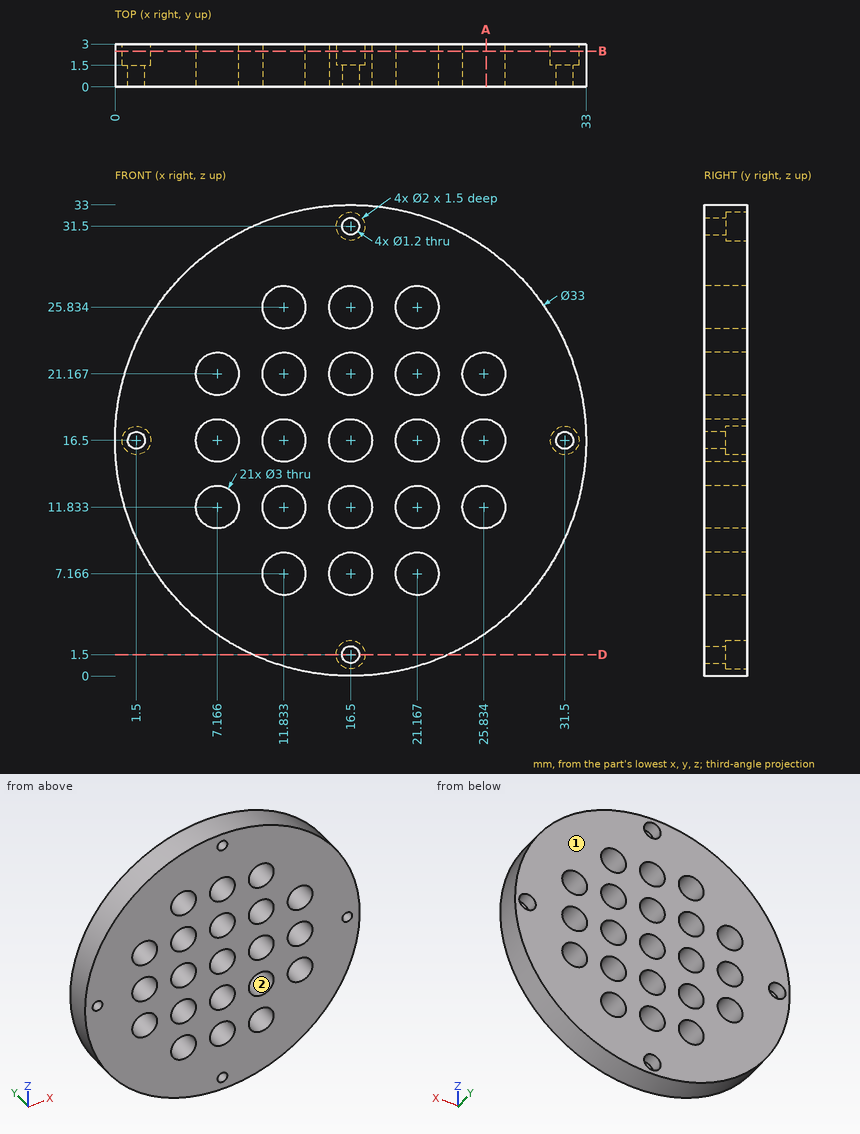
Here's the drawing with two shaded views (mm, measured from the low corner). I have some questions. Round coordinates to 2 decimals unless told otherwise and drop trailing zeros. Loops run counter-clockwise (first coordinate to the right, second up) from the corner with the lowest first, then second, coordinate; pieces in that order, holes last. Notation, with made-up numbers: M 88,-23.75 L 95,-23.75 A16 ccw 95,-0.75 Z; hole C 81,-3 d11. An arc over 180 degrees is marked long. Put each result on its own line as item: value.
Q1. Imagine slicing it at D-D (z = 1.5). Write out the boundary of the cut face in (x, y).
Check result:
outline: M 9.63,0 L 15.9,0 L 15.9,1.5 L 15.5,1.5 L 15.5,3 L 9.63,3 Z; M 17.1,0 L 23.37,0 L 23.37,3 L 17.5,3 L 17.5,1.5 L 17.1,1.5 Z
Q2. Imagine slicing it at B-B (y = 2.5). State how many separate pieces and enclosed holes the cut face has, then the cut area to 3 significant figures.
Check result:
separate pieces: 1
enclosed holes: 25
area: 694 mm2
Q3. Imagine slicing it at A-A (x = 26). Write out the boundary of the cut face in (y, z), then the cut area to 3 significant figures.
Check result:
outline: M 0,3.01 L 3,3.01 L 3,10.34 L 0,10.34 Z; M 0,13.32 L 3,13.32 L 3,15.01 L 0,15.01 Z; M 0,17.99 L 3,17.99 L 3,19.68 L 0,19.68 Z; M 0,22.66 L 3,22.66 L 3,29.99 L 0,29.99 Z
area: 54.1 mm2
Q4. For pin 1 (1.6 mm diameter, centred on x = 16.5, z = 31.5, fed in from +Y); pin 2 (1.5 mm diameter, centred on x = 11, y = 1, fed in from +Z); pin 3 (1 mm diameter, centred on y = 2, z = 12.5, fed in from -X), each with a flat end and sliding along its axis, tell me the tip position at first contact or that it passes through.
Check result:
pin 1: y = 1.5
pin 2: z = 32.3
pin 3: x = 0.38
Q5. I need wall thicknesses on probe 1 along X at (y, z) = (0.4, 7); probe 2 along X at (y, z) = (0.55, 8). Which ranges of each line are inside material? Lowest first, please.
Check result:
probe 1: 3.01 to 10.34, 13.32 to 15.01, 17.99 to 19.68, 22.66 to 29.99
probe 2: 2.36 to 10.59, 13.08 to 15.25, 17.75 to 19.92, 22.41 to 30.64
Q6. Thinking about a two-plate mould opening in X: for the marked faces 1 and 2, which applies, released by +X, released by -X, zero draft, split by the parting line, or undercut?
Check result:
face 1: zero draft
face 2: undercut
